Verification items for the finished model (mm, model axes). A direction names the side the tool comes from. Coordinates: 2 decimals unless noted, no trailing zeros. Loops run counter-clockwise (first coordinate to the right, second up) from the corner with the lowest first, then second, coordinate; pieces in that order, holes last. Notation, with made-up numbers: (70, 54.25) -> (106, 54.25) arc R3 ccw to (106, 58.25) -> close; hole circle Ø5 at (67, -23). An arc over 180 degrees is marked (long way). Write item = value, one per line.
```python
from build123d import *

# Parameters (mm, degrees)
BOSS_EXTRUDE1_DEPTH = 65
CHAMFER1_SIZE       = 10
SKETCH2_R           = 15
CUT_EXTRUDE1_DEPTH  = 5
SKETCH3_R           = 1.5
CUT_EXTRUDE2_DEPTH  = 7.5
FILLET1_R           = 1
SKETCH4_W           = 15
SKETCH4_H           = 40
CUT_EXTRUDE3_DEPTH  = 180.530638054
SKETCH5_R           = 1.5
SKETCH5_W           = 15
SKETCH5_H           = 27
CUT_EXTRUDE4_DEPTH  = 10


with BuildPart() as part:
    # Sketch1 → Boss-Extrude1 (new body)
    with BuildSketch(Plane.XY):
        with BuildLine():
            Line((-37.5, 162.5), (37.5, 162.5))
            Line((37.5, 162.5), (39.995249108, 0.616480975))
            ThreePointArc((39.995249108, 0.616480975), (0, -40), (-39.995249108, 0.616480975))
            Line((-39.995249108, 0.616480975), (-37.5, 162.5))
        make_face()
    extrude(amount=BOSS_EXTRUDE1_DEPTH)

    # Chamfer1
    chamfer1_edges = [part.edges().sort_by_distance(p)[0] for p in [
        (-38.747624554, 81.558240488, 65),
        (0, -40, 65),
        (38.747624554, 81.558240488, 65),
        (0, -40, 0),
        (-38.747624554, 81.558240488, 0),
        (38.747624554, 81.558240488, 0),
    ]]
    chamfer(chamfer1_edges, length=CHAMFER1_SIZE)

    # Sketch2 → Cut-Extrude1 (cut)
    with BuildSketch(Plane.XY.offset(65)):
        Circle(SKETCH2_R)
    extrude(amount=-CUT_EXTRUDE1_DEPTH, mode=Mode.SUBTRACT)

    # Sketch3 → Cut-Extrude2 (cut)
    with BuildSketch(Plane.XY.offset(60)):
        with Locations((0, 7.5)):
            Circle(SKETCH3_R)
        with Locations((7.5, 0)):
            Circle(SKETCH3_R)
        with Locations((0, -7.5)):
            Circle(SKETCH3_R)
        with Locations((-7.5, 0)):
            Circle(SKETCH3_R)
    extrude(amount=-CUT_EXTRUDE2_DEPTH, mode=Mode.SUBTRACT)

    # Fillet1
    fillet1_edges = [part.edges().sort_by_distance(p)[0] for p in [
        (-15, 0, 60),
        (-15, 0, 65),
    ]]
    fillet(fillet1_edges, radius=FILLET1_R)

    # Sketch4 → Cut-Extrude3 (cut, through all)
    with BuildSketch(Plane.XY.offset(65)):
        with Locations((0, 132.5)):
            Rectangle(SKETCH4_W, SKETCH4_H)
    extrude(amount=-CUT_EXTRUDE3_DEPTH, mode=Mode.SUBTRACT)

    # Sketch5 → Cut-Extrude4 (cut)
    with BuildSketch(Plane(origin=(0, 162.5, 0), x_dir=(1, 0, 0), z_dir=(0, 1, 0))):
        with Locations(Location((-3.25, -15.75, 0), (0, 0, 270))):
            Circle(SKETCH5_R)
        with Locations(Location((3.25, -15.75, 0), (0, 0, 270))):
            Circle(SKETCH5_R)
        with Locations(Location((3.25, -49.25, 0), (0, 0, 270))):
            Circle(SKETCH5_R)
        with Locations(Location((-3.25, -49.25, 0), (0, 0, 270))):
            Circle(SKETCH5_R)
        with Locations((0, -32.5)):
            Rectangle(SKETCH5_W, SKETCH5_H)
    extrude(amount=-CUT_EXTRUDE4_DEPTH, mode=Mode.SUBTRACT)


solid = part.part
```
1) Sectioned sample at A-A, the plane z = 35. Record the cut outline in (x, y).
Ans:
outline = (-40, 0.62) arc R40 ccw (long way) to (40, 0.62) -> (37.5, 162.5) -> (7.5, 162.5) -> (7.5, 112.5) -> (-7.5, 112.5) -> (-7.5, 162.5) -> (-37.5, 162.5) -> close
2) Release check for a two-part mould opening along X. For faces 5 (the face through (0, 68, 65)), 6 (the face through (0, 152.5, 10)), 7 (the face through (0.89, -39.99, 32.18)) record: pulls with the +X half, pulls with the -X half, needs draft (parallel to the pull), parting line crosses it, or undercut.
Ans:
face_5 = needs draft
face_6 = undercut
face_7 = parting line crosses it
3) Sectioned sample at B-B, the plane y = 43. Record the cut outline in (x, z).
Ans:
outline = (-39.34, 10) -> (-29.34, 0) -> (29.34, 0) -> (39.34, 10) -> (39.34, 55) -> (29.34, 65) -> (-29.34, 65) -> (-39.34, 55) -> close
4) Material ranges on line 1 (X direction, y = 157, z = 15); line 2 (Z direction, x = 3.5, y = -3.5); line 3 (Y direction, x = 7, z = 57), recorded low to high.
Ans:
line_1 = -37.58 to -4.55, -1.95 to 1.95, 4.55 to 37.58
line_2 = 0 to 60
line_3 = -37.35 to -1.41, 1.41 to 112.5, 152.5 to 162.5
5) Sectioned sample at C-C, the plane z = 57. Record the cut outline in (x, y), plus the area to 3 significant figures.
Ans:
outline = (-38, 0.59) arc R38 ccw (long way) to (38, 0.59) -> (35.5, 162.5) -> (-35.5, 162.5) -> close; hole circle Ø3 at (-7.5, 0); hole (-7.5, 112.5) -> (7.5, 112.5) -> (7.5, 152.5) -> (-7.5, 152.5) -> close; hole circle Ø3 at (0, -7.5); hole circle Ø3 at (0, 7.5); hole circle Ø3 at (7.5, 0)
area = 13,600 mm2
6) Sectioned sample at D-D, the plane z = 7. Record the cut outline in (x, y), plus the area to 3 significant figures.
Ans:
outline = (-37, 0.57) arc R37 ccw (long way) to (37, 0.57) -> (34.5, 162.5) -> (-34.5, 162.5) -> close; hole (-7.5, 112.5) -> (7.5, 112.5) -> (7.5, 152.5) -> (-7.5, 152.5) -> close
area = 13,200 mm2
7) Depth check by flat-ended pin: pin 1 Ø25 at (y, z) = (140.5, 36.5) entering from +X; pin 2 Ø0.9 at (x, y) = (7.5, 0) entering from +Z; pin 3 Ø4.5 at (x, z) = (-3, 14) entering from -Y. Enter the tip coordinate at first touch or a pass-through.
Ans:
pin_1 = 38.03
pin_2 = 52.5
pin_3 = -39.99
8) Tool access check on faces 1 (the face through (0, 158, 19)), 2 (the face through (0, 0, 60)), 3 (the face through (0, 68, 0)), 4 (the face through (0, 152.5, 56)). Record the directions out of +Z, -Z, +X, -X, +Y, -Y that give a thin tool (end or side, any length) a straight path to the whole face; none if there is none.
Ans:
face_1 = +Y
face_2 = +Z
face_3 = -Z, +X, -X, +Y, -Y
face_4 = +Z, -Z
